```python
from build123d import *

# Parameters (mm, degrees)
F0_R     = 11
F0_R_2   = 6
F0_R_3   = 4.025
F1_DEPTH = 2
F2_DEPTH = 0.6
F3_DEPTH = 3.6
F4_R     = 1
F5_SIZE  = 0.6


with BuildPart() as f1:
    # F0 (on Top) → F1 (new body)
    with BuildSketch(Plane.XY):
        Circle(F0_R)
        Circle(F0_R_2, mode=Mode.SUBTRACT)
        Circle(F0_R_2)
        Circle(F0_R_3, mode=Mode.SUBTRACT)
        Circle(F0_R_3)
    extrude(amount=-F1_DEPTH)

    # F0 (on Top) → F2 (join)
    with BuildSketch(Plane.XY):
        Circle(F0_R_2)
        Circle(F0_R_3, mode=Mode.SUBTRACT)
    extrude(amount=F2_DEPTH)

    # F0 (on Top) → F3 (join)
    with BuildSketch(Plane.XY):
        Circle(F0_R_3)
    extrude(amount=F3_DEPTH)

    # F4
    f4_edges = [f1.edges().sort_by_distance(p)[0] for p in [
        (-11, 0, -2),
    ]]
    fillet(f4_edges, radius=F4_R)

    # F5
    f5_edges = [f1.edges().sort_by_distance(p)[0] for p in [
        (-4.025, 0, 3.6),
    ]]
    chamfer(f5_edges, length=F5_SIZE)


solid = f1.part
```
Verification items for the finished model (mm, model axes). A direction names the side the tool comes from. Give positions to 0.01 mm unless a question says otherwise; leave off trailing zeros. Order: outer loops, then holes, each group sorted by start corner. A loop starts at its lowest first (then second) coordinate and runs counter-clockwise, first axis right, second up. Notation, with made-up numbers: M 74,88.5 L 99,88.5 A12 cw 99,97.5 Z; hole C 47,88.5 d6. An arc over 180 degrees is marked long. Return JSON: item names as keys, results as strings. Group by question number.
1) Mould release check, pull along X, two halves, no side actions. Record for faces 3 (the face through (0, 0, -2)), 4 (the face through (3.84, 1.21, 1.78)): pulls with the +X half, pulls with the -X half, needs draft (parallel to the pull), parting line crosses it, or undercut.
2) Section check C-C on z = -1.4. Record the cut outline in (x, y), and give its area (3 significant figures).
3) Go/stop test with a flat-tipped pin: pin 1 Ø1.5 at (y, z) = (-9, 0) entering from +X. Record where the tip stops, or that it passes through.
4) Scan lines: line 1 (Z direction, x = -6.25, y = 4); line 2 (Z direction, x = 3.25, y = -2.5); line 3 (Y direction, x = 3.75, z = -1.55). Record each from-to range of solid material in increasing order.
5) Section check A-A on x = 0. Record the cut outline in (y, z) (3 decimals), and give its area (3 significant figures).
6) Access from +Z, -Z, +X, -X, +Y, -Y to the whole of each face (thin tool, end or side, straight path). Record for faces 1 (the face through (5, -5, 0)), 2 (the face through (-2.38, -10.74, -0.49)).
7) Section check B-B on z = 2.2. Record the cut outline in (x, y) (3 decimals), and give its area (3 significant figures).
Answer block:
{
 "1": {"face 3": "needs draft", "face 4": "parting line crosses it"},
 "2": {"outline": "C 0,0 d21.83", "area": "374 mm^2"},
 "3": {"pin 1": "stops at x = 7.28"},
 "4": {"line 1": "z = -2 to 0", "line 2": "z = -2 to 0.6", "line 3": "y = -10.17 to 10.17"},
 "5": {"outline": "M -11,-1 A1 ccw -10,-2 L 10,-2 A1 ccw 11,-1 L 11,0 L 6,0 L 6,0.6 L 4.025,0.6 L 4.025,3 L 3.425,3.6 L -3.425,3.6 L -4.025,3 L -4.025,0.6 L -6,0.6 L -6,0 L -11,0 Z", "area": "74.6 mm^2"},
 "6": {"face 1": "+Z", "face 2": "+Z, -Z"},
 "7": {"outline": "C 0,0 d8.05", "area": "50.9 mm^2"}
}
